For this review, take the finished solid that the model builds, in its own axes (mm). Face numbers are marked on the shaded views. A direction names the side the tool comes from. Give positions to 0.01 mm unless a question says otherwise; leave off trailing zeros. Loops run counter-clockwise (first coordinate to the right, second up) from the corner with the lowest first, then second, coordinate; pieces in that order, holes last. Notation, with made-up numbers: (85.5, 74) - (116.5, 74) arc R14 ccw to (116.5, 95) - close; hole circle Ø8 at (80, -18.75). An arc over 180 degrees is marked (long way). Use CSV: the item, a comma, the result in double quotes. Start each with the question number.
1. Take a section at B-B on y = 10. Give the boundary of the cut face in (x, z), plus the area to 3 significant figures.
2. Take a section at C-C on y = 4.5. Give the boundary of the cut face in (x, z), plus the area to 3 significant figures.
3. Wall thickness on line 1 (Y direction, x = 16, z = 1.85); line 2 (X direction, y = 9.25, z = 10.75): over which ranges is each line inside the solid? List them lowest first.
4. Take a section at A-A on x = 16. Give the boundary of the cut face in (y, z).
5. Take a section at D-D on z = 19.25. Give the boundary of the cut face in (x, y), plus the area to 3 significant figures.
6. For pin 1 (9.5 mm diameter, centred on x = 15.5, y = 9, fed in from +Z); pin 2 (2 mm diameter, centred on y = 17, z = 9, fed in from +X); pin 3 (3 mm diameter, centred on y = 2.5, z = 8, fed in from +X), all flat-tipped, find the tip position at first contact; note any pin that passes through.
7. For the marked faces 1 and 2, list the 3-axis set-ups (+Z, -Z, +X, -X, +Y, -Y) from which the entire face can be reached by the end or side of a thin tool; tool diameter is ignored.
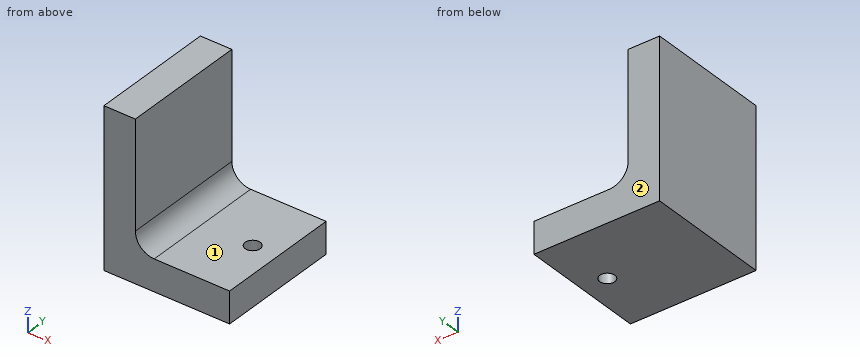
```python
from build123d import *

# Parameters (mm, degrees)
SKETCH1_W           = 20
SKETCH1_H           = 20
BOSS_EXTRUDE1_DEPTH = 5
SKETCH2_W           = 5
SKETCH2_H           = 20
BOSS_EXTRUDE2_DEPTH = 20
FILLET1_R           = 3
SKETCH3_R           = 1.2
CUT_EXTRUDE1_DEPTH  = 20


with BuildPart() as part:
    # Sketch1 → Boss-Extrude1 (new body)
    with BuildSketch(Plane.XY):
        with Locations((10, 10)):
            Rectangle(SKETCH1_W, SKETCH1_H)
    extrude(amount=BOSS_EXTRUDE1_DEPTH)

    # Sketch2 → Boss-Extrude2 (add)
    with BuildSketch(Plane.XY.offset(5)):
        with Locations((2.5, 10)):
            Rectangle(SKETCH2_W, SKETCH2_H)
    extrude(amount=BOSS_EXTRUDE2_DEPTH)

    # Fillet1
    fillet1_edges = [part.edges().sort_by_distance(p)[0] for p in [
        (5, 10, 5),
    ]]
    fillet(fillet1_edges, radius=FILLET1_R)

    # Sketch3 → Cut-Extrude1 (cut)
    with BuildSketch(Plane(origin=(0, 0, 0), x_dir=(-1, 0, 0), z_dir=(0, 0, -1))):
        with Locations((-16, 10)):
            Circle(SKETCH3_R)
    extrude(amount=-CUT_EXTRUDE1_DEPTH, mode=Mode.SUBTRACT)


solid = part.part
```
Check result:
1,outline,"(0, 0) - (14.8, 0) - (14.8, 5) - (8, 5) arc R3 cw to (5, 8) - (5, 25) - (0, 25) - close; (17.2, 0) - (20, 0) - (20, 5) - (17.2, 5) - close"
1,area,"190 mm²"
2,outline,"(0, 0) - (20, 0) - (20, 5) - (8, 5) arc R3 cw to (5, 8) - (5, 25) - (0, 25) - close"
2,area,"202 mm²"
3,line 1,"y = 0 to 8.8, 11.2 to 20"
3,line 2,"x = 0 to 5"
4,outline,"(0, 0) - (8.8, 0) - (8.8, 5) - (0, 5) - close; (11.2, 0) - (20, 0) - (20, 5) - (11.2, 5) - close"
5,outline,"(0, 0) - (5, 0) - (5, 20) - (0, 20) - close"
5,area,"100 mm²"
6,pin 1,"stops at z = 5"
6,pin 2,"stops at x = 5"
6,pin 3,"stops at x = 5.4"
7,face 1,"+Z, +X, +Y, -Y"
7,face 2,"+Z, -Z, +X, -X, +Y"
